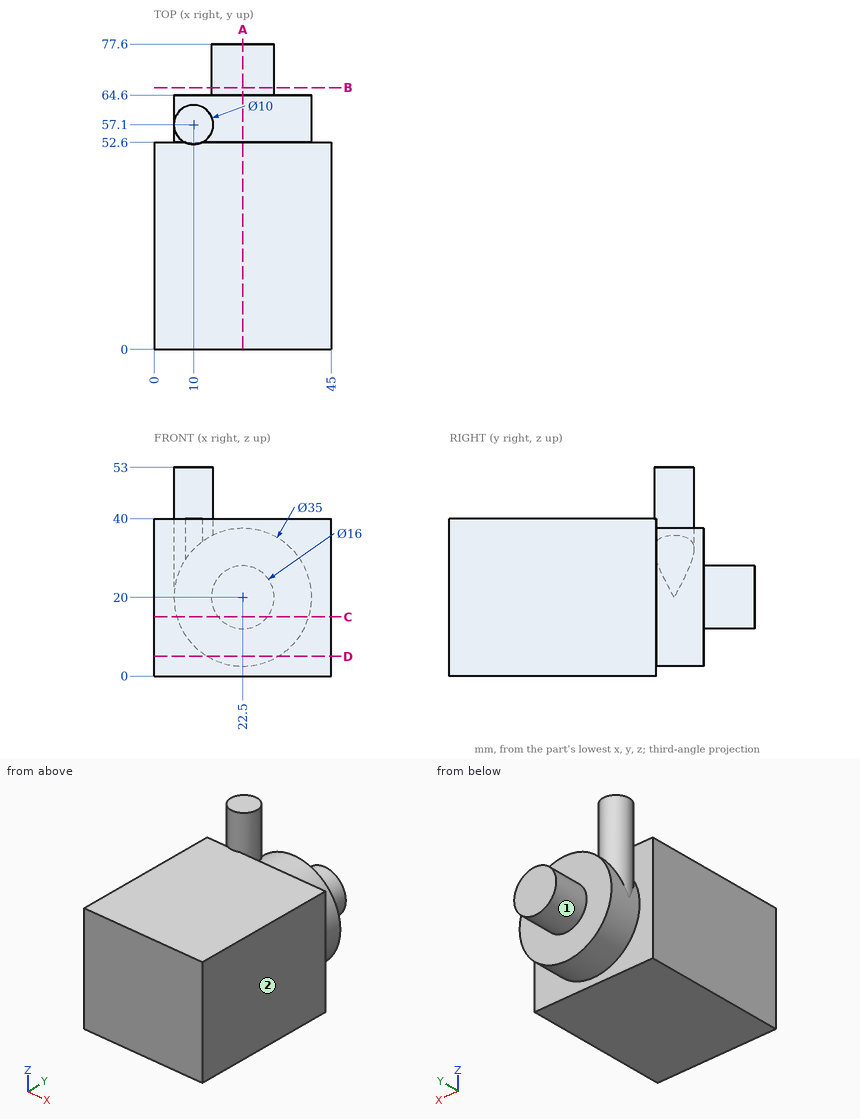
Part print with two shaded views. Sizes in mm from the minimum x, y, z corner. A direction names the side the tool comes from. Round coordinates to 2 decimals unless told otherwise and drop trailing zeros. Order: outer loops, then holes, each group sorted by start corner. A loop starts at its lowest first (then second) coordinate and runs counter-clockwise, first axis right, second up. Notation, with made-up numbers: (87, 36.5) - (123, 36.5) arc R19 cw to (123, 65.5) - close; hole circle Ø1 at (66, 51.25). An arc over 180 degrees is marked (long way). Return JSON: item names as keys, results as strings.
(1) Tool access for the marked faces 1 and 2: list every direction of +Z, -Z, +X, -X, +Y, -Y with a clear straight run to the whole face (end or side of a thin tool).
Answer key:
{"face 1": "+Y", "face 2": "+Z, -Z, +X, +Y, -Y"}
(2) Cut at C-C (z = 15). Give the cut face in (x, y) (1 decimal).
Answer key:
{"outline": "(0, 0) - (45, 0) - (45, 52.6) - (39.3, 52.6) - (39.3, 64.6) - (28.7, 64.6) - (28.7, 77.6) - (16.3, 77.6) - (16.3, 64.6) - (5.7, 64.6) - (5.7, 52.6) - (0, 52.6) - close"}
(3) Cut at A-A (x = 22.5). Give the cut face in (y, z), then the cut area to 3 significant figures.
Answer key:
{"outline": "(0, 0) - (52.6, 0) - (52.6, 2.5) - (64.6, 2.5) - (64.6, 12) - (77.6, 12) - (77.6, 28) - (64.6, 28) - (64.6, 37.5) - (52.6, 37.5) - (52.6, 40) - (0, 40) - close", "area": "2,730 mm^2"}
(4) Cut at D-D (z = 5). Give the cut face in (x, y), then the cut area to 3 significant figures.
Answer key:
{"outline": "(0, 0) - (45, 0) - (45, 52.6) - (31.51, 52.6) - (31.51, 64.6) - (13.49, 64.6) - (13.49, 52.6) - (0, 52.6) - close", "area": "2,580 mm^2"}
(5) Wall check: probe 1 along Z at (x, y) = (25, 8.5); probe 2 along Y at (x, z) = (23.5, 28); probe 3 along Y at (x, z) = (6, 39). Give the ranges that are in metal, low to high. Write a range as from..to.
Answer key:
{"probe 1": "z = 0..40", "probe 2": "y = 0..64.6", "probe 3": "y = 0..52.6, 54.1..60.1"}
(6) Pin check, flat tips, straight feed: pin 1 Ø8 at (x, y) = (31, 11) entering from +Z; pin 2 Ø1 at (x, y) = (12, 18) entering from -Z; pin 3 Ø10 at (y, z) = (66, 36) entering from +X. Stop position of each tip, or through.
Answer key:
{"pin 1": "stops at z = 40", "pin 2": "stops at z = 0", "pin 3": "stops at x = 35.95"}
(7) Cut at B-B (y = 66.5). Give the cut face in (x, z).
Answer key:
{"outline": "circle Ø16 at (22.5, 20)"}
